Build history of the part. All positions in model axes, mm. A direction names the side the tool comes from. Give positions to 0.01 mm unless a question says otherwise; leave off trailing zeros. Order: outer loops, then holes, each group sorted by start corner. A loop starts at its lowest first (then second) coordinate and runs counter-clockwise, first axis right, second up. Notation, with made-up numbers: (54.5, 25) - (100.5, 25) arc R37 cw to (100.5, 63) - close; hole circle Ø7 at (26.5, 86.25). An arc over 180 degrees is marked (long way). One line per item, written item: value.
```python
from build123d import *

# Parameters (mm, degrees)
SKETCH1_W           = 15
SKETCH1_H           = 500
SKETCH1_R           = 5
BOSS_EXTRUDE1_DEPTH = 10
SKETCH2_W           = 200
SKETCH2_H           = 100
BOSS_EXTRUDE2_DEPTH = 100


with BuildPart() as part:
    # Sketch1 → Boss-Extrude1 (new body)
    with BuildSketch(Plane.XY):
        with Locations((0, -240)):
            Rectangle(SKETCH1_W, SKETCH1_H)
        Circle(SKETCH1_R, mode=Mode.SUBTRACT)
    extrude(amount=BOSS_EXTRUDE1_DEPTH)

    # Sketch2 → Boss-Extrude2 (add)
    with BuildSketch(Plane.XZ.offset(490)):
        with Locations((-0.2, 5)):
            Rectangle(SKETCH2_W, SKETCH2_H)
    extrude(amount=BOSS_EXTRUDE2_DEPTH)


solid = part.part
```
(1) Slice it at A-A, the plane x = -71. Give the cut face in (y, z), and give its area (3 significant figures).
Completed:
outline: (-590, -45) - (-490, -45) - (-490, 55) - (-590, 55) - close
area: 10,000 mm²
(2) Pin check, flat tips, straight feed: P1, Ø6, axis at y = -211, z = 10, coming from the +X side; P2, Ø12, axis at x = 0, y = -245, coming from the +Z side; P3, Ø7.5, axis at x = 1.5, y = -278, coming from the -Z side. Stop position of each tip, or through.
Completed:
P1: x = 7.5
P2: z = 10
P3: z = 0
(3) Slice it at B-B, the plane y = -80. Give the cut face in (x, z), and give its area (3 significant figures).
Completed:
outline: (-7.5, 0) - (7.5, 0) - (7.5, 10) - (-7.5, 10) - close
area: 150 mm²
(4) Pull direction Y, two halves, no side cores. Call faces 1 (the face through (7.5, -243, 5)), 2 (the face through (-2, -590, 6)), 3 (the face through (-1.08, -4.88, 4.93)): +Y half, -Y half, draft (parallel to the pull), parting line (faces both ways), or undercut.
Completed:
face 1: draft
face 2: -Y half
face 3: undercut
(5) 3-axis set-ups, long thin cutter, end or side, ignore diameter. For faces 4 (the face through (0, -236, 10)), 5 (the face through (-7.5, -243, 5)), 6 (the face through (0, -236, 0)): which of +Z, -Z, +X, -X, +Y, -Y reach the whole face in a straight line?
Completed:
face 4: +Z, +X, -X, +Y
face 5: +Z, -Z, -X, +Y
face 6: -Z, +X, -X, +Y
(6) Drill centre lines: line 1 (Y direction, x = 0, z = 2.25); line 2 (X direction, y = -250, z = 7.5); line 3 (Y direction, x = -88.5, z = -33.5). Where is each one in solid material? Low to high.
Completed:
line 1: -590 to -5, 5 to 10
line 2: -7.5 to 7.5
line 3: -590 to -490
